Design review of the part built by this model. Coordinates are the model's own, in mm. A direction names the side the tool comes from. Coordinates: 2 decimals unless noted, no trailing zeros. Write each loop counter-clockwise with the first axis right and the second up, starting at its lowest first coordinate (ties: lowest second). Pieces come first, ordered by that corner, then holes.
Q1. Machinability: for faces 5 (the flat face through (20, 20, 3)), 6 (the cylindrical face through (46.974, 12.526, 3.131)), 7 (the flat face through (105, 20, 3)), which of the approach directions +Z, -Z, +X, -X, +Y, -Y give a long, thin tool a straight path to every point of the face, cutting with its end or side? Answer none if there is none.
Q2. For probe 1 along X at (y, z) = (27, 4.5); probe 2 along X at (y, z) = (13.5, 3.75); probe 3 along Y at (x, z) = (75, 2.5), list the stretches that pass through material, from the lowest coordinate up.
Q3. Take a section at C-C (y = 40). Give the boundary of the cut face in (x, z).
Q4. Take a section at B-B (x = 115). Give the boundary of the cut face in (y, z), and give its area (3 significant figures).
Q5. Take a section at A-A (y = 20). Give the boundary of the cut face in (x, z).
Q6. Insertion check: pin 1 (3 mm diameter, centred on y = 25, z = 4.5, fed in from -X); pin 2 (1.9 mm diameter, centred on y = 23, z = 4.5, fed in from +X). Each pin has a flat end and moves straight along its axis. Give the tip position at first contact, or say it passes through.
Q7. Take a section at D-D (z = 3.25). State how many separate pieces and enclosed holes the cut face has, and give its area (3 significant figures).
Q8. Mouldability with a two-part tool opening along Y and no side actions: class faces 1 (the flat face through (76, 31, 6.35)), 2 (the cylindrical face through (73.123, 15.595, 3.219)), 3 (the cylindrical face through (117.027, 41.859, 3.131)), 4 (the flat face through (62, 0, 3)) as pulls with the +Y half, pulls with the -Y half, needs draft (parallel to the pull), parting line crosses it, or undercut.
```python
from build123d import *

# Parameters (mm, degrees)
SKETCH1_W           = 125
SKETCH1_H           = 50
BOSS_EXTRUDE1_DEPTH = 6.35
SKETCH2_R           = 11.5
CUT_EXTRUDE1_DEPTH  = 7.35
SKETCH5_R           = 1.75
CUT_EXTRUDE5_DEPTH  = 7.35
SKETCH6_R           = 2.75
SKETCH6_W           = 20
SKETCH6_H           = 30
CUT_EXTRUDE6_DEPTH  = 7.35
FILLET1_R           = 10


with BuildPart() as part:
    # Sketch1 → Boss-Extrude1 (new body)
    with BuildSketch(Plane.XY):
        with Locations((62.5, 25)):
            Rectangle(SKETCH1_W, SKETCH1_H)
    extrude(amount=BOSS_EXTRUDE1_DEPTH)

    # Sketch2 → Cut-Extrude1 (cut, through all)
    with BuildSketch(Plane.XY.offset(6.35)):
        with Locations((62.5, 20)):
            Circle(SKETCH2_R)
    extrude(amount=-CUT_EXTRUDE1_DEPTH, mode=Mode.SUBTRACT)

    # Sketch5 → Cut-Extrude5 (cut, through all)
    with BuildSketch(Plane(origin=(0, 0, 0), x_dir=(-1, 0, 0), z_dir=(0, 0, -1))):
        with Locations((-48.643593539, 28)):
            Circle(SKETCH5_R)
        with Locations((-48.643593539, 12)):
            Circle(SKETCH5_R)
        with Locations((-62.5, 4)):
            Circle(SKETCH5_R)
        with Locations((-76.356406461, 12)):
            Circle(SKETCH5_R)
        with Locations((-76.356406461, 28)):
            Circle(SKETCH5_R)
        with Locations((-62.5, 36)):
            Circle(SKETCH5_R)
    extrude(amount=-CUT_EXTRUDE5_DEPTH, mode=Mode.SUBTRACT)

    # Sketch6 → Cut-Extrude6 (cut, through all)
    with BuildSketch(Plane(origin=(0, 0, 0), x_dir=(-1, 0, 0), z_dir=(0, 0, -1))):
        with Locations((-115, 40)):
            Circle(SKETCH6_R)
        with Locations((-10, 40)):
            Circle(SKETCH6_R)
        with Locations((-115, 15)):
            Rectangle(SKETCH6_W, SKETCH6_H)
        with Locations((-10, 15)):
            Rectangle(SKETCH6_W, SKETCH6_H)
    extrude(amount=-CUT_EXTRUDE6_DEPTH, mode=Mode.SUBTRACT)

    # Fillet1
    fillet1_edges = [part.edges().sort_by_distance(p)[0] for p in [
        (105, 0, 3.175),
        (20, 0, 3.175),
    ]]
    fillet(fillet1_edges, radius=FILLET1_R)


solid = part.part
```
Response:
1. face 5: +Z, -Z, -X, -Y
1. face 6: +Z, -Z
1. face 7: +Z, -Z, +X, -Y
2. probe 1: x = 20 to 47.21, 50.08 to 53.38, 71.62 to 74.92, 77.79 to 105
2. probe 2: x = 20 to 47.74, 49.54 to 53.01, 71.99 to 75.46, 77.26 to 105
2. probe 3: y = 0 to 10.89, 13.11 to 26.89, 29.11 to 50
3. outline: (0, 0) - (7.25, 0) - (7.25, 6.35) - (0, 6.35) - close; (12.75, 0) - (112.25, 0) - (112.25, 6.35) - (12.75, 6.35) - close; (117.75, 0) - (125, 0) - (125, 6.35) - (117.75, 6.35) - close
4. outline: (30, 0) - (37.25, 0) - (37.25, 6.35) - (30, 6.35) - close; (42.75, 0) - (50, 0) - (50, 6.35) - (42.75, 6.35) - close
4. area: 92.1 mm2
5. outline: (20, 0) - (51, 0) - (51, 6.35) - (20, 6.35) - close; (74, 0) - (105, 0) - (105, 6.35) - (74, 6.35) - close
6. pin 1: stops at x = 20
6. pin 2: stops at x = 105
7. separate pieces: 1
7. enclosed holes: 9
7. area: 4,490 mm2
8. face 1: needs draft
8. face 2: undercut
8. face 3: undercut
8. face 4: pulls with the -Y half
